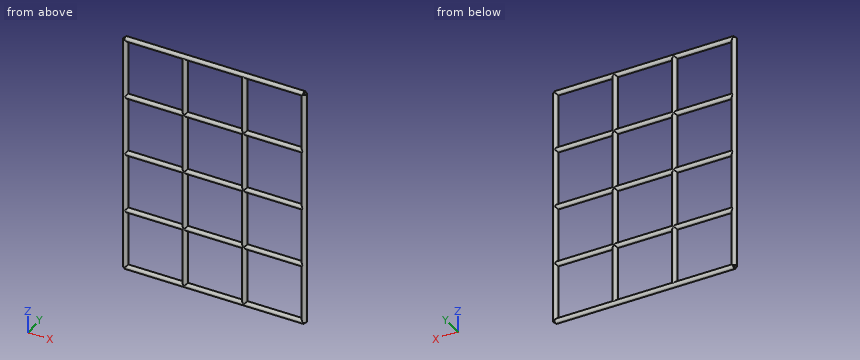
from build123d import *

# Parameters (mm, degrees)
SKETCH1_R           = 1.9812
BASE_EXTRUDE_DEPTH  = 203.2
SKETCH2_R           = 1.9812
BOSS_EXTRUDE1_DEPTH = 152.4
LPATTERN1_START     = -203.2
LPATTERN1_OUTLINE_R = 1.9812
LPATTERN1_DEPTH     = 203.2
LPATTERN2_COUNT     = 5
LPATTERN2_PITCH     = 50.8


# Read off the part's stored shape, not the designer's step: LPattern1
with BuildPart() as part:
    # Sketch1 → Base-Extrude (new body)
    with BuildSketch(Plane.XY):
        Circle(SKETCH1_R)
    extrude(amount=-BASE_EXTRUDE_DEPTH)

    # Sketch2 → Boss-Extrude1 (add)
    with BuildSketch(Plane(origin=(0, 0, 0), x_dir=(0, 0, -1), z_dir=(1, 0, 0))):
        Circle(SKETCH2_R)
    boss_extrude1 = extrude(amount=BOSS_EXTRUDE1_DEPTH)

    # LPattern1 outline → LPattern1 (add)
    with BuildSketch(Plane.XY.offset(LPATTERN1_START)):
        with Locations((50.8, 0)):
            Circle(LPATTERN1_OUTLINE_R)
        with Locations((101.6, 0)):
            Circle(LPATTERN1_OUTLINE_R)
        with Locations((152.4, 0)):
            Circle(LPATTERN1_OUTLINE_R)
    extrude(amount=LPATTERN1_DEPTH)

    # LPattern2: Boss-Extrude1 ×5
    with Locations(*[(0, 0, -i * LPATTERN2_PITCH) for i in range(1, LPATTERN2_COUNT)]):
        add(boss_extrude1)


solid = part.part
Source: CAD feature listing. Evaluate the final solid. Frame: model axes, mm. Give positions to 0.01 mm unless a question says otherwise; leave off trailing zeros. Write each loop counter-clockwise with the first axis right and the second up, starting at its lowest first coordinate (ties: lowest second). Pieces come first, ordered by that corner, then holes. Notation, with made-up numbers: (77, 79.5) -> (106, 79.5) arc R13 ccw to (106, 86.5) -> close; hole circle Ø6 at (-18, -6.75). An arc over 180 degrees is marked (long way). Return JSON: item names as keys, results as strings. Group by question number.
1. Section C-C, the plane y = 0. Count the separate pieces of the cut face and the enclosed holes in it, then the cut area to 3 significant figures.
2. Material intervals for line 1 (Z direction, x = 40.5, y = -0.1); line 2 (X direction, y = -0.1, z = -67); line 3 (X direction, y = 0.5, z = -85.5), sorted ascending. Write a range as from..to.
3. Section A-A, the plane x = 93. Output: boundary loops of the cut face in (y, z), then the cut area to 3 significant figures.
4. Pin query (flat end, axial travel): pin 1 Ø12 at (x, z) = (72, -59) entering from -Y; pin 2 Ø2 at (x, y) = (154, 1) entering from +Z; pin 3 Ø2 at (y, z) = (0, -204.5) entering from -X; pin 4 Ø2 at (x, y) = (154, 0) entering from -Z. Return the tip coordinate at first contact, or that it passes through.
5. Section B-B, the plane z = -174.5. Output: boundary loops of the cut face in (x, y), then the cut area to 3 significant figures.
Determined:
{
 "1": {"separate pieces": "1", "enclosed holes": "12", "area": "6,050 mm2"},
 "2": {"line 1": "z = -205.18..-201.22, -154.38..-150.42, -103.58..-99.62, -52.78..-48.82, -1.98..1.98", "line 2": "x = -1.98..1.98, 48.82..52.78, 99.62..103.58, 150.42..154.38", "line 3": "x = -1.92..1.92, 48.88..52.72, 99.68..103.52, 150.48..154.32"},
 "3": {"outline": "circle Ø3.96 at (0, -203.2); circle Ø3.96 at (0, -152.4); circle Ø3.96 at (0, -101.6); circle Ø3.96 at (0, -50.8); circle Ø3.96 at (0, 0)", "area": "61.7 mm2"},
 "4": {"pin 1": "passes through", "pin 2": "stops at z = 0", "pin 3": "stops at x = 0", "pin 4": "stops at z = -203.2"},
 "5": {"outline": "circle Ø3.96 at (0, 0); circle Ø3.96 at (50.8, 0); circle Ø3.96 at (101.6, 0); circle Ø3.96 at (152.4, 0)", "area": "49.3 mm2"}
}
